Build history of the part. All positions in model axes, mm. A direction names the side the tool comes from. Give positions to 0.01 mm unless a question says otherwise; leave off trailing zeros. Order: outer loops, then holes, each group sorted by start corner. A loop starts at its lowest first (then second) coordinate and runs counter-clockwise, first axis right, second up. Notation, with made-up numbers: (50, -32.75) - (93, -32.75) arc R18 cw to (93, -17.75) - close; hole circle Ø2 at (20, -23.5). An arc over 180 degrees is marked (long way). Use a Markdown table: item, result.
from build123d import *

# Parameters (mm, degrees)
CHAMFER1_SIZE = 1
FILLET1_R     = 0.5


with BuildPart() as part:
    # Sketch1 → Revolve1 (revolve)
    with BuildSketch(Plane.XY):
        Polygon((-10, 1.5), (-10, 3.175), (0, 3.175), (0, 5.175), (4, 5.175), (4, 3.175), (9, 3.175), (9, 1.5), align=None)
    revolve(axis=Axis((-34.824359623, 0, 0), (1, 0, 0)))

    # Chamfer1
    chamfer1_edges = [part.edges().sort_by_distance(p)[0] for p in [
        (-10, -3.175, 0),
    ]]
    chamfer(chamfer1_edges, length=CHAMFER1_SIZE)

    # Fillet1
    fillet1_edges = [part.edges().sort_by_distance(p)[0] for p in [
        (0, -5.175, 0),
        (4, -5.175, 0),
    ]]
    fillet(fillet1_edges, radius=FILLET1_R)


solid = part.part
1) Wall check: line 1 (Z direction, x = 0.5, y = 0) (3 decimals); line 2 (Z direction, x = -4.5, y = 0) (3 decimals); line 3 (Y direction, x = -3.25, z = 0.25). Give the ranges that are in metal, low to high. Write a range as from..to.
Computed:
| item | result |
|---|---|
| line 1 | z = -5.175..-1.5, 1.5..5.175 |
| line 2 | z = -3.175..-1.5, 1.5..3.175 |
| line 3 | y = -3.17..-1.48, 1.48..3.17 |
2) Slice it at A-A (z = 0). Write the cut outline in (x, y) (3 decimals).
Computed:
| item | result |
|---|---|
| outline | (-10, -2.175) - (-9, -3.175) - (0, -3.175) - (0, -4.675) arc R0.5 ccw to (0.5, -5.175) - (3.5, -5.175) arc R0.5 ccw to (4, -4.675) - (4, -3.175) - (9, -3.175) - (9, -1.5) - (-10, -1.5) - close; (-10, 1.5) - (9, 1.5) - (9, 3.175) - (4, 3.175) - (4, 4.675) arc R0.5 ccw to (3.5, 5.175) - (0.5, 5.175) arc R0.5 ccw to (0, 4.675) - (0, 3.175) - (-9, 3.175) - (-10, 2.175) - close |
3) Slice it at C-C (x = -3). Write the cut outline in (y, z) (3 decimals), and give its area (3 significant figures).
Computed:
| item | result |
|---|---|
| outline | circle Ø6.35 at (0, 0); hole circle Ø3 at (0, 0) |
| area | 24.6 mm² |
4) Two-plate mould, pull along Y, no slides. Class faces 3 (the cylindrical face through (-4.44, -0.69, -3.1)), 4 (the cylindrical face through (-0.63, -1.5, 0.07)), 5 (the flat face through (9, 0.7, 1.5)): +Y half, -Y half, draft (parallel to the pull), parting line (faces both ways), or undercut.
Computed:
| item | result |
|---|---|
| face 3 | parting line |
| face 4 | undercut |
| face 5 | draft |
5) Tool access for faces 1 (the cylindrical face through (6.54, -0.69, -3.1)), 2 (the cylindrical face through (2.021, -4.107, -3.149)): list every direction of +Z, -Z, +X, -X, +Y, -Y with a clear straight run to the whole face (end or side of a thin tool).
Computed:
| item | result |
|---|---|
| face 1 | +X |
| face 2 | +X, -X |
6) Pin check, flat tips, straight feed: P1, Ø2, axis at x = -6, y = 3.5, coming from the +Z side; P2, Ø6, axis at x = -4.5, y = 0.5, coming from the -Z side (3 decimals); P3, Ø4, axis at x = -4.5, z = 2.5, coming from the -Y side; P4, Ø2.5, axis at y = 0, z = 0, coming from the +X side. Stop position of each tip, or through.
Computed:
| item | result |
|---|---|
| P1 | stops at z = 1.96 |
| P2 | stops at z = -3.175 |
| P3 | stops at y = -3.14 |
| P4 | passes through |
